from build123d import *

# Parameters (mm, degrees)
BOSS_EXTRUDE1_DEPTH = 50.8
BOSS_EXTRUDE2_START = -7.62
SKETCH1_3_W         = 48.1
SKETCH1_3_H         = 50.8
SKETCH1_3_R         = 2.5
BOSS_EXTRUDE2_DEPTH = 7.62
SKETCH2_R           = 1.5
CUT_EXTRUDE1_DEPTH  = 12.7
SKETCH3_R           = 1.5
CUT_EXTRUDE2_DEPTH  = 12.7
FILLET1_R           = 12.7


with BuildPart() as part:
    # Sketch1 → Boss-Extrude1 (new body)
    with BuildSketch(Plane(origin=(0, 0, 0), x_dir=(1, 0, 0), z_dir=(0, 1, 0))):
        with BuildLine():
            Line((3.592102448, -3.592102448), (37.527491057, 30.34328616))
            Line((37.527491057, 30.34328616), (42.915644729, 24.955132487))
            Line((42.915644729, 24.955132487), (8.980256121, -8.980256121))
            ThreePointArc((8.980256121, -8.980256121), (0, -12.7), (-8.980256121, -8.980256121))
            ThreePointArc((-8.980256121, -8.980256121), (-27.044794722, -5.28871851), (-37.527491057, -20.45671384))
            Line((-37.527491057, -20.45671384), (-45.147491057, -20.45671384))
            Line((-45.147491057, -20.45671384), (-45.147491057, 30.34328616))
            Line((-45.147491057, 30.34328616), (-37.527491057, 30.34328616))
            Line((-37.527491057, 30.34328616), (-3.592102448, -3.592102448))
            ThreePointArc((-3.592102448, -3.592102448), (0, -5.08), (3.592102448, -3.592102448))
        make_face()
    extrude(amount=BOSS_EXTRUDE1_DEPTH)

    # Sketch1_3 → Boss-Extrude2 (add)
    # profile 1 of 3: a face of its own
    with BuildSketch(Plane(origin=(0, 0, 0), x_dir=(1, 0, 0), z_dir=(0, 1, 0)).offset(BOSS_EXTRUDE2_START)):
        with BuildLine():
            ThreePointArc((-3.592102448, -3.592102448), (0, -5.08), (3.592102448, -3.592102448))
            Line((3.592102448, -3.592102448), (20.559796753, 13.375591856))
            Line((20.559796753, 13.375591856), (-20.559796753, 13.375591856))
            Line((-20.559796753, 13.375591856), (-3.592102448, -3.592102448))
        make_face()
    # profile 2 of 3: a face of its own
    with BuildSketch(Plane(origin=(0, 0, 0), x_dir=(1, 0, 0), z_dir=(0, 1, 0)).offset(BOSS_EXTRUDE2_START)):
        with BuildLine():
            Line((20.559796753, 13.375591856), (3.592102448, -3.592102448))
            ThreePointArc((3.592102448, -3.592102448), (0, -5.08), (-3.592102448, -3.592102448))
            Line((-3.592102448, -3.592102448), (-20.559796753, 13.375591856))
            Line((-20.559796753, 13.375591856), (-37.527491057, 30.34328616))
            Line((-37.527491057, 30.34328616), (-45.147491057, 30.34328616))
            Line((-45.147491057, 30.34328616), (-45.147491057, -20.45671384))
            Line((-45.147491057, -20.45671384), (-37.527491057, -20.45671384))
            ThreePointArc((-37.527491057, -20.45671384), (-27.044794722, -5.28871851), (-8.980256121, -8.980256121))
            ThreePointArc((-8.980256121, -8.980256121), (0, -12.7), (8.980256121, -8.980256121))
            Line((8.980256121, -8.980256121), (42.915644729, 24.955132487))
            Line((42.915644729, 24.955132487), (37.527491057, 30.34328616))
            Line((37.527491057, 30.34328616), (20.559796753, 13.375591856))
        make_face()
    # profile 3 of 3: a face of its own
    with BuildSketch(Plane(origin=(0, 0, 0), x_dir=(1, 0, 0), z_dir=(0, 1, 0)).offset(BOSS_EXTRUDE2_START)):
        with Locations((-69.197491057, 4.94328616)):
            Rectangle(SKETCH1_3_W, SKETCH1_3_H)
        with Locations(Location((-83.247491057, -7.75671384, 0), (0, 0, 270))):
            Circle(SKETCH1_3_R, mode=Mode.SUBTRACT)
        with Locations(Location((-83.247491057, 17.64328616, 0), (0, 0, 270))):
            Circle(SKETCH1_3_R, mode=Mode.SUBTRACT)
    extrude(amount=BOSS_EXTRUDE2_DEPTH)

    # Sketch2 → Cut-Extrude1 (cut)
    with BuildSketch(Plane(origin=(-3.592102448, 0, 3.592102448), x_dir=(-0.7071067811865488, 0, -0.7071067811865464), z_dir=(0.7071067811865464, 0, -0.7071067811865488))):
        with Locations((22.591886814, 38.1)):
            Circle(SKETCH2_R)
        with Locations((22.591886814, 11.43)):
            Circle(SKETCH2_R)
    extrude(amount=-CUT_EXTRUDE1_DEPTH, mode=Mode.SUBTRACT)

    # Sketch3 → Cut-Extrude2 (cut)
    with BuildSketch(Plane(origin=(3.592102448, 0, 3.592102448), x_dir=(-0.7071067811865488, 0, 0.7071067811865464), z_dir=(-0.7071067811865464, 0, -0.7071067811865488))):
        with Locations((-22.591886814, 38.1)):
            Circle(SKETCH3_R)
        with Locations((-22.591886814, 11.43)):
            Circle(SKETCH3_R)
    extrude(amount=-CUT_EXTRUDE2_DEPTH, mode=Mode.SUBTRACT)

    # Fillet1
    fillet1_edges = [part.edges().sort_by_distance(p)[0] for p in [
        (-45.147491057, 0, -4.94328616),
    ]]
    fillet(fillet1_edges, radius=FILLET1_R)


solid = part.part
Verification items for the finished model (mm, model axes). A direction names the side the tool comes from. Coordinates: 2 decimals unless noted, no trailing zeros. Order: outer loops, then holes, each group sorted by start corner. A loop starts at its lowest first (then second) coordinate and runs counter-clockwise, first axis right, second up. Notation, with made-up numbers: M 74,-17 L 117,-17 A24 ccw 117,1 Z; hole C -12.75,64 d6. An arc over 180 degrees is marked long. Return JSON: item names as keys, results as strings.
1) Cross-section at A-A, the plane y = 46. Record the boundary of the cut face in (x, z), and give its area (3 significant figures).
Answer list:
{"outline": "M -45.15,-30.34 L -37.53,-30.34 L -3.59,3.59 A5.08 cw 3.59,3.59 L 37.53,-30.34 L 42.92,-24.96 L 8.98,8.98 A12.7 ccw -8.98,8.98 A16.72 cw -37.53,20.46 L -45.15,20.46 Z", "area": "1,540 mm2"}
2) Gauge pin test, flat ends, axial feed: pin 1 (12 mm diameter, centred on x = -15.5, y = 14, fed in from -Z); pin 2 (12 mm diameter, centred on x = -7.5, y = 15.5, fed in from -Z); pin 3 (9 mm diameter, centred on x = 7, z = -3, fed in from +Y); pin 4 (3 mm diameter, centred on x = -53.5, z = 8.5, fed in from +Y). Record the tip position at first contact, or that the pin passes through.
Answer list:
{"pin 1": "z = -14.32", "pin 2": "z = -6.32", "pin 3": "y = 50.8", "pin 4": "y = 1.43"}
3) Release check for a two-part mould opening along X. For faces 1 (the flat face through (-76, 0, -5)), 2 (the cylindrical face through (-23.856, 39.587, -7.817)), 3 (the flat face through (25.71, 21.18, -7.75)), 4 (the flat face through (-45.147, 31, -5)) record: +X half, -X half, draft (parallel to the pull), parting line (faces both ways), or undercut.
Answer list:
{"face 1": "draft", "face 2": "undercut", "face 3": "+X half", "face 4": "-X half"}
4) Thickness scan on L1, parallel to X at y = 7, z = -18; L2, parallel to X at y = 37, z = 2.5; L3, parallel to Y at x = -81.5, z = 12. Record the ranges inside material, lowest first. Write a range as [from, to].
Answer list:
{"L1": "[-46.5, -25.18], [25.18, 35.96]", "L2": "[-45.15, -4.68], [4.68, 15.46]", "L3": "[-7.62, 0]"}
5) Cross-section at D-D, the plane z = 14. Record the boundary of the cut face in (x, y).
Answer list:
{"outline": "M -93.25,-7.62 L -36.08,-7.62 L -36.08,50.8 L -45.15,50.8 L -45.15,12.7 A12.7 cw -57.85,0 L -93.25,0 Z"}
6) Cross-section at C-C, the plane z = -23. Record the boundary of the cut face in (x, y), and give its area (3 significant figures).
Answer list:
{"outline": "M -93.25,-7.62 L -30.18,-7.62 L -30.18,50.8 L -45.15,50.8 L -45.15,12.7 A12.7 cw -57.85,0 L -93.25,0 Z; M 30.18,-7.62 L 40.96,-7.62 L 40.96,50.8 L 30.18,50.8 Z", "area": "1,900 mm2"}
7) Access from +Z, -Z, +X, -X, +Y, -Y to the whole of each face (thin tool, end or side, straight path). Record for faces 5 (the flat face through (40.26, 21.18, -27.61)), 6 (the flat face through (0, 0, -6)), 7 (the flat face through (0, -4, -13.376)).
Answer list:
{"face 5": "-Z, +X, +Y, -Y", "face 6": "-Z, +Y", "face 7": "-Z, +Y, -Y"}
8) Cross-section at B-B, the plane y = -3. Record the boundary of the cut face in (x, z).
Answer list:
{"outline": "M -93.25,-30.34 L -37.53,-30.34 L -20.56,-13.38 L 20.56,-13.38 L 37.53,-30.34 L 42.92,-24.96 L 8.98,8.98 A12.7 ccw -8.98,8.98 A16.72 cw -37.53,20.46 L -93.25,20.46 Z; hole C -83.25,-17.64 d5; hole C -83.25,7.76 d5"}
